Source: CAD feature listing. Evaluate the final solid. Frame: model axes, mm. A direction names the side the tool comes from. Coordinates: 2 decimals unless noted, no trailing zeros. Order: outer loops, then holes, each group sorted by start corner. A loop starts at its lowest first (then second) coordinate and runs counter-clockwise, first axis right, second up.
```python
from build123d import *

# Parameters (mm, degrees)
Y_KSEKLIK_EKSTR_ZYON1_DEPTH = 12
IZIM3_R                     = 3.15
KES_EKSTR_ZYON1_DEPTH       = 61.745370194
KES_EKSTR_ZYON2_DEPTH       = 2
KES_EKSTR_ZYON5_REACH       = 62.745
IZIM8_R                     = 3.75
KES_EKSTR_ZYON3_REACH       = 61.481
IZIM6_R                     = 0.5
KES_EKSTR_ZYON4_DEPTH       = 21
RADYUS1_R                   = 5
FILLET1_R                   = 5
CUT_EXTRUDE2_DEPTH          = 10


with BuildPart() as part:
    # Çizim2 → Yükseklik-Ekstrüzyon1 (new body)
    with BuildSketch(Plane(origin=(0, 0, 0), x_dir=(1, 0, 0), z_dir=(0, 1, 0))):
        with BuildLine():
            Line((-45, -15.5), (-45, -20.5))
            Line((-45, -20.5), (-10, -20.5))
            Line((-10, -20.5), (-6.022579038, -7.5))
            Line((-6.022579038, -7.5), (0, -7.5))
            Line((0, -7.5), (0, 7.5))
            Line((0, 7.5), (-6.022579038, 7.5))
            Line((-6.022579038, 7.5), (-10, 18.5))
            Line((-10, 18.5), (-45, 18.5))
            Line((-45, 18.5), (-45, 15.5))
            Line((-45, 15.5), (-20, 15.5))
            ThreePointArc((-20, 15.5), (-16.464466094, 14.035533906), (-15, 10.5))
            Line((-15, 10.5), (-15, -10.5))
            ThreePointArc((-15, -10.5), (-16.464466094, -14.035533906), (-20, -15.5))
            Line((-20, -15.5), (-45, -15.5))
        make_face()
    y_kseklik_ekstr_zyon1 = extrude(amount=Y_KSEKLIK_EKSTR_ZYON1_DEPTH)

    # Çizim3 → Kes-Ekstrüzyon1 (cut, through all)
    with BuildSketch(Plane.XY.offset(20.5)):
        with Locations((-38, 6)):
            Circle(IZIM3_R)
    kes_ekstr_zyon1 = extrude(amount=-KES_EKSTR_ZYON1_DEPTH, mode=Mode.SUBTRACT)

    # Çizim5 → Kes-Ekstrüzyon2 (cut)
    with BuildSketch(Plane.XY.offset(20.5)):
        with BuildLine():
            ThreePointArc((-34.25, 6), (-35.1875, 3.519608146), (-37.53125, 2.279412219))
            Line((-37.53125, 2.279412219), (-23.75, 4.015686517))
            ThreePointArc((-23.75, 4.015686517), (-22, 6), (-23.75, 7.984313483))
            Line((-23.75, 7.984313483), (-37.53125, 9.720587781))
            ThreePointArc((-37.53125, 9.720587781), (-35.1875, 8.480391854), (-34.25, 6))
        make_face()
    kes_ekstr_zyon2 = extrude(amount=-KES_EKSTR_ZYON2_DEPTH, mode=Mode.SUBTRACT)

    # Çizim8 → Kes-Ekstrüzyon5 (cut, up to next)
    with BuildSketch(Plane.XY.offset(20.5), mode=Mode.PRIVATE) as kes_ekstr_zyon5_sk1:
        with Locations((-38, 6)):
            Circle(IZIM8_R)
    kes_ekstr_zyon5_tool1 = extrude(kes_ekstr_zyon5_sk1.sketch, amount=-KES_EKSTR_ZYON5_REACH, mode=Mode.PRIVATE) & part.part
    kes_ekstr_zyon5 = kes_ekstr_zyon5_tool1.solids().sort_by_distance((-38, 6, 20.5))[0]
    add(kes_ekstr_zyon5, mode=Mode.SUBTRACT)

    # Çizim6 → Kes-Ekstrüzyon3 (cut, up to next)
    with BuildSketch(Plane.XY.offset(18.5), mode=Mode.PRIVATE) as kes_ekstr_zyon3_sk1:
        with Locations((-26, 6)):
            Circle(IZIM6_R)
    kes_ekstr_zyon3_tool1 = extrude(kes_ekstr_zyon3_sk1.sketch, amount=-KES_EKSTR_ZYON3_REACH, mode=Mode.PRIVATE) & part.part
    kes_ekstr_zyon3 = kes_ekstr_zyon3_tool1.solids().sort_by_distance((-26, 6, 18.5))[0]
    add(kes_ekstr_zyon3, mode=Mode.SUBTRACT)

    # Aynalama1: Yükseklik-Ekstrüzyon1, Kes-Ekstrüzyon1, Kes-Ekstrüzyon2, Kes-Ekstrüzyon5, Kes-Ekstrüzyon3 across plane
    add(y_kseklik_ekstr_zyon1.mirror(Plane(origin=(0, 12, -7.5), x_dir=(0, 0, 1), z_dir=(-1, 0, 0))))
    add(kes_ekstr_zyon1.mirror(Plane(origin=(0, 12, -7.5), x_dir=(0, 0, 1), z_dir=(-1, 0, 0))), mode=Mode.SUBTRACT)
    add(kes_ekstr_zyon2.mirror(Plane(origin=(0, 12, -7.5), x_dir=(0, 0, 1), z_dir=(-1, 0, 0))), mode=Mode.SUBTRACT)
    add(kes_ekstr_zyon5.mirror(Plane(origin=(0, 12, -7.5), x_dir=(0, 0, 1), z_dir=(-1, 0, 0))), mode=Mode.SUBTRACT)
    add(kes_ekstr_zyon3.mirror(Plane(origin=(0, 12, -7.5), x_dir=(0, 0, 1), z_dir=(-1, 0, 0))), mode=Mode.SUBTRACT)

    # Çizim7 → Kes-Ekstrüzyon4 (cut, symmetric)
    with BuildSketch(Plane.XY):
        with BuildLine():
            Line((-12.5, 6.5), (12.5, 6.5))
            ThreePointArc((12.5, 6.5), (19, 0), (12.5, -6.5))
            Line((12.5, -6.5), (-12.5, -6.5))
            ThreePointArc((-12.5, -6.5), (-19, 0), (-12.5, 6.5))
        make_face()
    extrude(amount=KES_EKSTR_ZYON4_DEPTH, both=True, mode=Mode.SUBTRACT)

    # Radyus1
    radyus1_edges = [part.edges().sort_by_distance(p)[0] for p in [
        (-45, 0, -17),
        (-19, 0, 17.949489743),
        (-19, 0, -16.949489743),
        (19, 0, 17.949489743),
        (19, 0, -16.949489743),
        (-45, 0, 18),
        (-45, 12, -17),
        (-45, 12, 18),
        (45, 12, -17),
        (45, 12, 18),
        (45, 0, 18),
        (45, 0, -17),
    ]]
    fillet(radyus1_edges, radius=RADYUS1_R)

    # Fillet1
    fillet1_edges = [part.edges().sort_by_distance(p)[0] for p in [
        (10, 9.25, 20.5),
        (6.022579038, 9.25, 7.5),
        (-10, 9.25, 20.5),
        (-6.022579038, 9.25, 7.5),
        (10, 9.25, -18.5),
        (6.022579038, 9.25, -7.5),
        (-10, 9.25, -18.5),
        (-6.022579038, 9.25, -7.5),
    ]]
    fillet(fillet1_edges, radius=FILLET1_R)

    # Sketch2 → Cut-Extrude2 (cut)
    with BuildSketch(Plane(origin=(0, 12, 0), x_dir=(1, 0, 0), z_dir=(0, 1, 0))):
        with BuildLine():
            Line((8.5, -1.9), (-8.5, -1.9))
            ThreePointArc((-8.5, -1.9), (-10.4, 0), (-8.5, 1.9))
            Line((-8.5, 1.9), (8.5, 1.9))
            ThreePointArc((8.5, 1.9), (10.4, 0), (8.5, -1.9))
        make_face()
    extrude(amount=-CUT_EXTRUDE2_DEPTH, mode=Mode.SUBTRACT)


solid = part.part
```
1. Ray query, line 1 (Y direction, x = -38, z = -17.8); line 2 (Z direction, x = 32, y = 2.25); line 3 (Y direction, x = 26, z = 16.2). Return the intervals inside material, ascending.
Findings:
line 1: y = 0 to 2.85, 9.15 to 12
line 2: z = -18.5 to -15.5, 15.5 to 20.5
line 3: y = 0 to 5.5, 6.5 to 12
2. Section query A-A on z = 0. Return loops of the section in (x, y), plus the area to 3 significant figures.
Findings:
outline: (-15, 6) arc R6.5 cw to (-12.5, 6.5) - (-10.4, 6.5) - (-10.4, 12) - (-15, 12) - close; (10.4, 6.5) - (12.5, 6.5) arc R6.5 cw to (15, 6) - (15, 12) - (10.4, 12) - close
area: 51.4 mm2
3. Section query C-C on x = 39. Return loops of the section in (y, z).
Findings:
outline: (0, -18.5) - (3.01, -18.5) - (3.01, -15.5) - (0, -15.5) - close; (0, 15.5) - (2.39, 15.5) - (2.39, 20.5) - (0, 20.5) - close; (8.99, -18.5) - (12, -18.5) - (12, -15.5) - (8.99, -15.5) - close; (9.61, 15.5) - (12, 15.5) - (12, 20.5) - (9.61, 20.5) - close
4. Access query for faces 1 (the face through (0, 9, -1.9)), 2 (the face through (30.737, 3.135, 19.514)), 3 (the face through (-20.16, 0.79, -16.84)), 4 (the face through (-10.7, 9.2, 19.5)). Directions: +Z, -Z, +X, -X, +Y, -Y. A direction counts if a zero-diameter tool reaches every point of the face in a straight line with its end or side. Return the directions, or none.
Findings:
face 1: +Y, -Y
face 2: +Z
face 3: +Z, -Z, -Y
face 4: +Z, +Y, -Y
5. Pin query (flat end, axial travel): P1, Ø3.5, axis at x = 31, y = 7, coming from the +Z side; P2, Ø6, axis at x = 3.5, y = 9, coming from the +Z side; P3, Ø7, axis at x = -38, y = 6, coming from the +Z side. Return the tip coordinate at first contact, or that it passes through.
Findings:
P1: stops at z = 18.5
P2: stops at z = 9.75
P3: stops at z = -15.5
6. Section query D-D on x = -32. Return loops of the section in (y, z), plus the area to 3 significant figures.
Findings:
outline: (0, -18.5) - (12, -18.5) - (12, -15.5) - (0, -15.5) - close; (0, 15.5) - (12, 15.5) - (12, 20.5) - (9.02, 20.5) - (9.02, 18.5) - (2.98, 18.5) - (2.98, 20.5) - (0, 20.5) - close
area: 83.9 mm2
7. Section query B-B on x = -4.5. Return loops of the section in (y, z), plus the area to 3 significant figures.
Findings:
outline: (6.5, -7.91) - (12, -7.91) - (12, -1.9) - (6.5, -1.9) - close; (6.5, 1.9) - (12, 1.9) - (12, 8) - (6.5, 8) - close
area: 66.6 mm2
8. Draft query along Z for faces 5 (the face through (29, 6, -18.5)), 6 (the face through (10.4, 9.3, 0)), 7 (the face through (-30.54, 8.84, 19.51)). Return one class per face: released by +Z, released by -Z, zero draft, split by the parting line, or undercut.
Findings:
face 5: released by -Z
face 6: undercut
face 7: zero draft
